Check sheet for the modelled part. Datum: model origin and axes. Units: mm. Give positions to 0.01 mm unless a question says otherwise; leave off trailing zeros. Order: outer loops, then holes, each group sorted by start corner. A loop starts at its lowest first (then second) coordinate and runs counter-clockwise, first axis right, second up. Notation, with made-up numbers: (41, 33) - (49, 33) arc R24 ccw to (49, 45) - close; hole circle Ø10 at (-1, 37). An arc over 180 degrees is marked (long way). Answer in a Markdown table with one row per item.
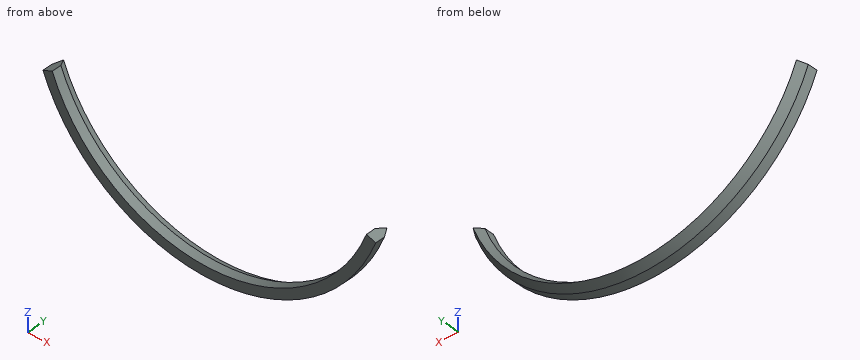
from build123d import *


with BuildPart() as part:
    # Sweep1: sweep along a path in PropShadow
    with BuildLine(Plane(origin=(0, 0, 0), x_dir=(1, 0, 0), z_dir=(0, 1, 0))) as sweep1_path:
        ThreePointArc((39.25, 15.138227876), (0, 42.068140478), (-39.25, 15.138227876))
    # Sketch4 → Sweep1 (sweep)
    with BuildSketch(Plane(origin=(0, 0, 0), x_dir=(0.9330101010986988, 0, 0.3598501788908768), z_dir=(-0.3598501788908768, 0, 0.9330101010986988))):
        Polygon((-43.268140478, 1.2), (-42.068140478, 3.2), (-40.868140478, 1.2), (-40.868140478, -1.2), (-43.268140478, -1.2), align=None)
    sweep(path=sweep1_path.line)


solid = part.part
(1) Cross-section at A-A, the plane y = 0.1. Record the cut outline in (x, z).
Geometry says:
| item | result |
|---|---|
| outline | (-40.37, -15.57) arc R43.27 ccw to (40.37, -15.57) - (38.13, -14.71) arc R40.87 cw to (-38.13, -14.71) - close |
(2) Gauge pin test, flat ends, axial feed: P1, Ø10, axis at x = 7.5, z = -34.5, coming from the -Y side; P2, Ø1.5, axis at y = -0.5, z = -40, coming from the +X side; P3, Ø1.5, axis at x = -20.5, y = 0.5, coming from the +Z side. Record the tip position at first contact, or that the pin passes through.
Geometry says:
| item | result |
|---|---|
| P1 | through |
| P2 | x = 18.21 |
| P3 | z = -34.91 |
(3) Thickness scan on L1, parallel to X at y = 0.4, z = -19.75; L2, parallel to X at y = 1.8, z = -38; L3, parallel to Y at x = -10, z = -41.25. Record the ranges inside material, lowest first.
Geometry says:
| item | result |
|---|---|
| L1 | -38.5 to -35.78, 35.78 to 38.5 |
| L2 | -19.93 to -15.99, 15.99 to 19.93 |
| L3 | -1.2 to 2.57 |
